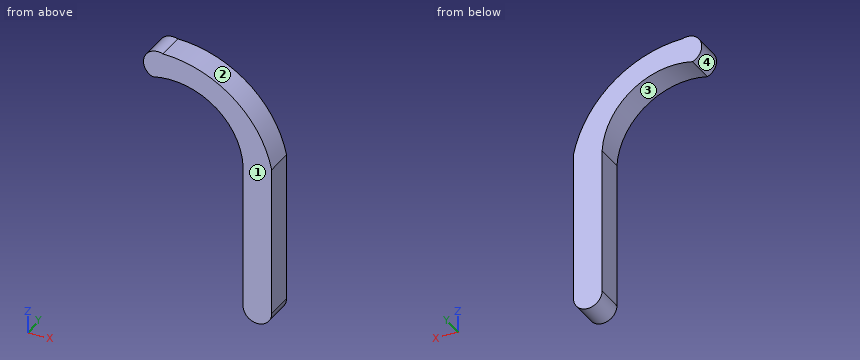
Autodesk Inventor part; units mm, degrees
ref_plane "YZ Plane" through (0, 0, 0) normal (1, 0, 0) x (0, 1, 0)
ref_plane "XZ Plane" through (0, 0, 0) normal (0, 1, 0) x (-1, 0, 0)
ref_plane "XY Plane" through (0, 0, 0) normal (0, 0, 1) x (1, 0, 0)
sketch "Sketch1" plane through (0, 0, 0) normal (0, 1, 0) x (-1, 0, 0)
  line L0 (0, 0) -> (0, 21) construction
  line L1 (-2, 0) -> (-2, 21)
  line L2 (2, 21) -> (2, 0)
  arc A0 (-2, 0) -> (2, 0) centre (0, 0) ccw
  arc A1 (2, 21) -> (-2, 21) centre (0, 21) ccw construction
  line L3 (0, 21) -> (4, 27.9282) construction
  line L4 (1.7321, 20) -> (5.7321, 26.9282) construction
  line L5 (2.2679, 28.9282) -> (-1.7321, 22) construction
  arc A2 (-1.7321, 22) -> (1.7321, 20) centre (0, 21) ccw construction
  arc A3 (5.7321, 26.9282) -> (2.2679, 28.9282) centre (4, 27.9282) ccw construction
  line L6 (4, 27.9282) -> (13.9336, 31.7413) construction
  line L7 (3.4527, 25.5758) -> (14.6503, 29.8742) construction
  line L8 (13.2168, 33.6085) -> (3.2833, 29.7954) construction
  arc A4 (3.2833, 29.7954) -> (3, 26.1962) centre (4, 27.9282) ccw construction
  arc A5 (14.6503, 29.8742) -> (13.2168, 33.6085) centre (13.9336, 31.7413) ccw
  line L9 (13.9336, 31.7413) -> (22.9322, 31.8984) construction
  arc A6 (13.2168, 33.6085) -> (-2, 21) centre (13.5169, 17.7597) ccw
  arc A7 (14.6503, 29.8742) -> (2, 20.4641) centre (12.3124, 19.8089) ccw
  point P0 (0, 10.5)
  point P1 (2, 24.4641)
  point P2 (-1.7321, 22)
  point P3 (8.9668, 29.8348)
  point P4 (5.3779, 26.3149)
  point P5 (18.4329, 31.8199)
  dimension "d0" = 4
  dimension "d5" = 25
  dimension "d6" = 150
  dimension "d7" = 4
  dimension "d8" = 12
  dimension "d9" = 12
  dimension "d10" = 111
  dimension "d11" = 200
  dimension "d13" = 9
extrude "Extrusion1" add sketch "Sketch1" along normal blind 4
equation "\"d7\" = d0"
properties part number "_3DPrint"
Input: part model. Units: mm. Frame: model coordinates. Face numbers are marked on the shaded views. Round coordinates to 2 decimals unless told otherwise and drop trailing zeros. Loops run counter-clockwise (first coordinate to the right, second up) from the corner with the lowest first, then second, coordinate; pieces in that order, holes last. Notation, with made-up numbers: (84.25, 47) -> (143.25, 47) arc R21 ccw to (143.25, 77) -> close; hole circle Ø5 at (-14, -0.75). An arc over 180 degrees is marked (long way). Answer as a JSON object with one key per item and string values. Group by question number.
1) Section query C-C on x = -2.75. Output: boundary loops of the cut face in (y, z).
2) Section query B-B on z = 7. Output: boundary loops of the cut face in (x, y).
3) Pin query (flat end, axial travel): pin 1 (2 mm diameter, centred on x = -5, y = 3.5, fed in from +Z); pin 2 (2 mm diameter, centred on x = -3.5, y = 1, fed in from +Z); pin 3 (1.5 mm diameter, centred on y = 2.5, z = 16.5, fed in from -X); pin 4 (4 mm diameter, centred on x = -6, z = 23, fed in from -Y). Return the tip coordinate at first contact, or that it passes through.
4) Draft query along X for the marked faces 1, 2, 3 and 4. Return one class per face: +X half, -X half, draft (parallel to the pull), parting line (faces both ways), or undercut.
5) Ray query, L1, parallel to X at y = 2.95, z = 11.5; L2, parallel to Z at x = -9.5, y = 2.4; L3, parallel to Z at x = -14.25, y = 0.95. Return the intervals inside material, ascending.
6) Section query A-A on y = 3.1. Output: boundary loops of the cut face in (x, z), plus the area to 3 significant figures.
Reply:
{
 "1": {"outline": "(0, 23.73) -> (4, 23.73) -> (4, 29.39) -> (0, 29.39) -> close"},
 "2": {"outline": "(-2, 0) -> (2, 0) -> (2, 4) -> (-2, 4) -> close"},
 "3": {"pin 1": "stops at z = 31.72", "pin 2": "stops at z = 30.8", "pin 3": "stops at x = -2", "pin 4": "passes through"},
 "4": {"face 1": "draft", "face 2": "+X half", "face 3": "undercut", "face 4": "parting line"},
 "5": {"L1": "x = -2 to 2", "L2": "z = 29.75 to 33.09", "L3": "z = 29.96 to 33.72"},
 "6": {"outline": "(-14.65, 29.87) arc R10.33 cw to (-2, 20.46) -> (-2, 0) arc R2 ccw to (2, 0) -> (2, 21) arc R15.85 ccw to (-13.22, 33.61) arc R2 ccw to start", "area": "162 mm2"}
}
